from build123d import *

# Parameters (mm, degrees)
F0_R     = 6.95
F0_R_2   = 6
F0_R_3   = 4.875
F0_R_4   = 2.5
F1_DEPTH = 1
F2_START = 1
F2_DEPTH = 7
F3_START = 8
F3_DEPTH = 1
F4_START = 9
F4_DEPTH = 7
F6_D     = 3.2
F6_DEPTH = 6.951


with BuildPart() as f1:
    # F0 (on Top) → F1 (new body)
    with BuildSketch(Plane.XY):
        Circle(F0_R)
        Circle(F0_R_2, mode=Mode.SUBTRACT)
        Circle(F0_R_2)
        Circle(F0_R_3, mode=Mode.SUBTRACT)
        Circle(F0_R_3)
        Circle(F0_R_4, mode=Mode.SUBTRACT)
    extrude(amount=F1_DEPTH)

    # F0 (on Top) → F2 (join)
    with BuildSketch(Plane.XY.offset(F2_START)):
        Circle(F0_R_2)
        Circle(F0_R_3, mode=Mode.SUBTRACT)
        Circle(F0_R_3)
        Circle(F0_R_4, mode=Mode.SUBTRACT)
    extrude(amount=F2_DEPTH)

    # F0 (on Top) → F3 (join)
    with BuildSketch(Plane.XY.offset(F3_START)):
        Circle(F0_R)
        Circle(F0_R_2, mode=Mode.SUBTRACT)
        Circle(F0_R_2)
        Circle(F0_R_3, mode=Mode.SUBTRACT)
        Circle(F0_R_3)
        Circle(F0_R_4, mode=Mode.SUBTRACT)
    extrude(amount=F3_DEPTH)

    # F0 (on Top) → F4 (join)
    with BuildSketch(Plane.XY.offset(F4_START)):
        Circle(F0_R)
        Circle(F0_R_2, mode=Mode.SUBTRACT)
        Circle(F0_R_2)
        Circle(F0_R_3, mode=Mode.SUBTRACT)
        Circle(F0_R_3)
        Circle(F0_R_4, mode=Mode.SUBTRACT)
    extrude(amount=F4_DEPTH)

    # F6 (through all, one way)
    with BuildSketch(Plane(origin=(0, 0, 0), x_dir=(0, 1, 0), z_dir=(-1, 0, 0))):
        with Locations((0, -12)):
            Circle(F6_D / 2)
    extrude(amount=-F6_DEPTH, mode=Mode.SUBTRACT)


solid = f1.part
Here's how the part is built. I have some questions about the finished solid (model axes, mm). A direction names the side the tool comes from. Coordinates: 2 decimals unless noted, no trailing zeros. Loops run counter-clockwise (first coordinate to the right, second up) from the corner with the lowest first, then second, coordinate; pieces in that order, holes last.
1. Imagine slicing it at C-C, the plane z = 9.5. Please give me the cut outline in (x, y), and give its area (3 significant figures).
2. Imagine slicing it at D-D, the plane x = 4.75. Please give me the cut outline in (y, z).
3. Imagine slicing it at B-B, the plane y = 0.25. Please give me the cut outline in (x, z), and give its area (3 significant figures).
4. For faces 1 (the cylindrical face through (4.4, -0.35, 13.56)), 2 (the flat face through (3, 0, 16)), 3 (the flat face through (-6, -2, 1)), which set-ups out of +Z, -Z, +X, -X, +Y, -Y let a thin tool reach every point of the face, with its end or its side?
5. If we mould it in two halves opening along X, with no side actions, what happens to faces 4 (the cylindrical face through (-1.507, -6.785, 11.944)), 5 (the cylindrical face through (-2.5, 0.1, 7.9)), 6 (the flat face through (3, 0, 0))? For each: pulls with the +X half, pulls with the -X half, needs draft (parallel to the pull), parting line crosses it, or undercut.
6. I need wall thicknesses on L1, parallel to Z at x = 2, y = 6.25; L2, parallel to Z at x = 5.15, y = 0; L3, parallel to Y at x = 0, z = 4. Which ranges of each line are inside material? Lowest first, please.
7. For P1, Ø3, axis at y = -2.5, z = 9, coming from the -X side; P2, Ø1.5, axis at x = -5, z = 2, coming from the +Y side; P3, Ø8, axis at x = 3.5, z = 5, coming from the -Y side, each with a flat end and sliding along its axis, tell me the tip position at first contact or that it passes through.
8. Imagine slicing it at A-A, the plane x = 0. Please give me the cut outline in (y, z).
Taken from the geometry:
1. outline: circle Ø13.9 at (0, 0); hole circle Ø5 at (0, 0)
1. area: 132 mm2
2. outline: (-5.07, 0) - (5.07, 0) - (5.07, 1) - (3.67, 1) - (3.67, 8) - (5.07, 8) - (5.07, 16) - (-5.07, 16) - (-5.07, 8) - (-3.67, 8) - (-3.67, 1) - (-5.07, 1) - close; hole circle Ø3.2 at (0, 12)
3. outline: (-6.95, 0) - (-2.49, 0) - (-2.49, 16) - (-6.95, 16) - (-6.95, 8) - (-5.99, 8) - (-5.99, 1) - (-6.95, 1) - close; (2.49, 0) - (6.95, 0) - (6.95, 1) - (5.99, 1) - (5.99, 8) - (6.95, 8) - (6.95, 10.42) - (2.49, 10.42) - close; (2.49, 13.58) - (6.95, 13.58) - (6.95, 16) - (2.49, 16) - close
3. area: 115 mm2
4. face 1: +X
4. face 2: +Z, +X, -X, +Y, -Y
4. face 3: none
5. face 4: parting line crosses it
5. face 5: undercut
5. face 6: needs draft
6. L1: z = 0 to 1, 8 to 16
6. L2: z = 0 to 10.4, 13.6 to 16
6. L3: y = -6 to -2.5, 2.5 to 6
7. P1: stops at x = -6.88
7. P2: stops at y = 4.24
7. P3: stops at y = -6.9
8. outline: (-6.95, 0) - (-2.5, 0) - (-2.5, 16) - (-6.95, 16) - (-6.95, 8) - (-6, 8) - (-6, 1) - (-6.95, 1) - close; (2.5, 0) - (6.95, 0) - (6.95, 1) - (6, 1) - (6, 8) - (6.95, 8) - (6.95, 16) - (2.5, 16) - close
